Could you check a few things on this drawing? It's one solid part, dimensions in mm from its lowest x, y, z. A direction names the side the tool comes from. Give positions to 0.01 mm unless a question says otherwise; leave off trailing zeros. Loops run counter-clockwise (first coordinate to the right, second up) from the corner with the lowest first, then second, coordinate; pieces in that order, holes last. Notation, with made-up numbers: M 89.25,44.25 L 110.25,44.25 A36 ccw 110.25,80.25 Z; hole C 65.25,21.25 d6. An arc over 180 degrees is marked long. Answer as a JSON object with one key per item and string values.
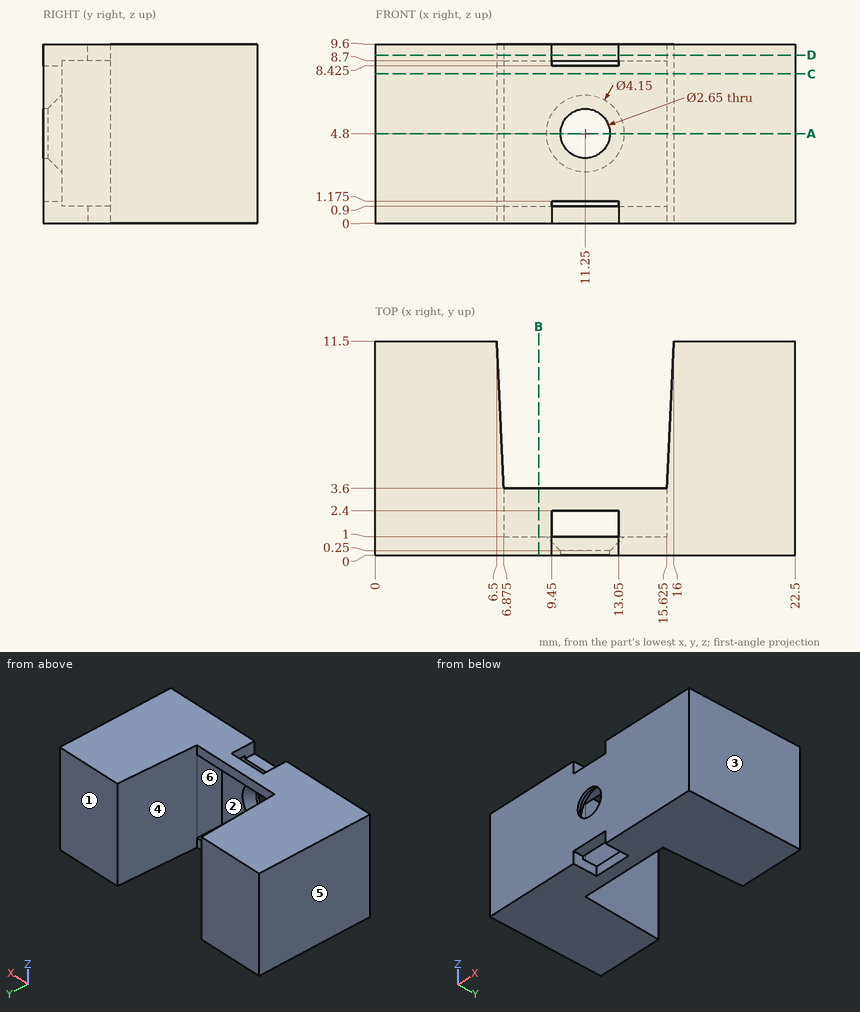
1) Suppose I cut it at B-B, the plane x = 8.75. Write out the boundary of the cut face in (y, z).
Answer list:
{"outline": "M 0,0 L 3.6,0 L 3.6,0.9 L 1,0.9 L 1,8.7 L 3.6,8.7 L 3.6,9.6 L 0,9.6 Z"}
2) Suppose I cut it at D-D, the plane z = 9. Write out the boundary of the cut face in (x, y) (3 decimals), and give its area (3 significant figures).
Answer list:
{"outline": "M 0,0 L 9.45,0 L 9.45,2.4 L 13.05,2.4 L 13.05,0 L 22.5,0 L 22.5,11.5 L 16,11.5 L 15.625,3.6 L 6.875,3.6 L 6.5,11.5 L 0,11.5 Z", "area": "178 mm^2"}
3) Suppose I cut it at C-C, the plane z = 8. Write out the boundary of the cut face in (x, y) (3 decimals).
Answer list:
{"outline": "M 0,0 L 22.5,0 L 22.5,11.5 L 16,11.5 L 15.625,3.6 L 15.625,1 L 6.875,1 L 6.875,3.6 L 6.5,11.5 L 0,11.5 Z"}
4) Please list where these lines run through material, in increasing order: line 1 along X through (y, z) = (0.1, 4.8) (3 decimals); line 2 along X through (y, z) = (2, 2) (3 decimals); line 3 along Y through (x, z) = (9, 7). Write a range as from..to.
Answer list:
{"line 1": "0..9.925, 12.575..22.5", "line 2": "0..6.875, 15.625..22.5", "line 3": "0..1"}
5) If we mould it in two halves opening along X, with no side actions, what happens to the marked faces 1, 2 and 3? For each: +X half, -X half, draft (parallel to the pull), parting line (faces both ways), or undercut.
Answer list:
{"face 1": "draft", "face 2": "undercut", "face 3": "+X half"}
6) Will these pins go through, and if not, where does the flat tip stop? pin 1 Ø0.7 at (x, z) = (11.5, 9.5) entering from -Y; pin 2 Ø0.5 at (x, y) = (10.5, 0.5) entering from -Z (3 decimals); pin 3 Ø2.5 at (x, z) = (11.25, 4.8) entering from +Y; pin 4 Ø2 at (x, z) = (8.5, 5) entering from +Y.
Answer list:
{"pin 1": "y = 2.4", "pin 2": "z = 1.175", "pin 3": "through", "pin 4": "y = 1"}
7) Suppose I cut it at A-A, the plane z = 4.8. Write out the boundary of the cut face in (x, y) (3 decimals), and give its area (3 significant figures).
Answer list:
{"outline": "M 0,0 L 9.925,0 L 9.925,0.25 L 9.175,1 L 6.875,1 L 6.875,3.6 L 6.5,11.5 L 0,11.5 Z; M 12.575,0 L 22.5,0 L 22.5,11.5 L 16,11.5 L 15.625,3.6 L 15.625,1 L 13.325,1 L 12.575,0.25 Z", "area": "161 mm^2"}
8) For the marked faces 4, 5 and 6, which set-ups out of +Z, -Z, +X, -X, +Y, -Y let a thin tool reach every point of the face, with its end or its side?
Answer list:
{"face 4": "+Z, -Z, +Y", "face 5": "+Z, -Z, -X, +Y, -Y", "face 6": "+Y"}
